Could you check a few things on this model? Use its own coordinates, in mm. Coordinates: 2 decimals unless noted, no trailing zeros. Write each loop counter-clockwise with the first axis right and the second up, starting at its lowest first coordinate (ties: lowest second). Pieces come first, ordered by that corner, then holes. Notation, with made-up numbers: M 10,-37.75 L 40,-37.75 A34 cw 40,-1.75 Z; hole C -15,-18.75 d8. An arc over 180 degrees is marked long. Answer as CSV lines item,"result". Start each with the question number.
Item 1: We'd pull the mould along X, two halves only. Please class faces 1 (the flat face through (212, 0, -68)), 2 (the cylindrical face through (355.283, 1.014, -88.32)): +X half, -X half, draft (parallel to the pull), parting line (faces both ways), or undercut.
Item 2: If I drill on line 1 along Z through (x, y) = (423, 1.1); line 2 along X through (y, z) = (0.7, -59); line 3 along Z through (x, y) = (338, 0.25), over which ranges is the centre line in solid material (lowest first)? Write a range as [from, to].
Item 3: Suppose I cut it at D-D, the plane x = 391. Write out the boundary of the cut face in (y, z), and give its area (3 significant figures).
Item 4: I'm going to push flat-ended pins straight in: P1, Ø6.5, axis at x = 7, z = -59, coming from the -Y side; P2, Ø1, axis at x = 5.5, y = 1, coming from the -Z side; P3, Ø0.6, axis at y = 1.5, z = -126.5, coming from the +X side; P4, Ø0.6, axis at x = 16.5, y = 1, coming from the +Z side. Where does each tip first touch, or does it pass through?
Item 5: Suppose I cut it at B-B, the plane z = -101. Write out the boundary of the cut face in (x, y).
Item 6: Suppose I cut it at C-C, the plane y = 0.4. Write out the boundary of the cut face in (x, z), and give its area (3 significant figures).
Item 7: Suppose I cut it at A-A, the plane x = 330. Write out the boundary of the cut face in (y, z).
```python
from build123d import *

# Parameters (mm, degrees)
SKETCH_2_W          = 430
SKETCH_2_H          = 135
EXTRUDE_1_DEPTH     = 2
SKETCH_3_R          = 2.5
SKETCH_3_W          = 12
SKETCH_3_H          = 15
SKETCH_3_W_2        = 60
SKETCH_3_H_2        = 30
CUT_EXTRUDE_1_DEPTH = 451.698347013
SKETCH_4_R          = 25.5
CUT_EXTRUDE_2_DEPTH = 451.698347013


with BuildPart() as part:
    # Эскиз2 → Бобышка-Вытянуть1 (new body)
    with BuildSketch(Plane(origin=(0, 0, 0), x_dir=(1, 0, 0), z_dir=(0, 1, 0))):
        with Locations((215, 67.5)):
            Rectangle(SKETCH_2_W, SKETCH_2_H)
    extrude(amount=EXTRUDE_1_DEPTH)

    # Эскиз3 → Вырез-Вытянуть1 (cut, through all)
    with BuildSketch(Plane(origin=(0, 2, 0), x_dir=(1, 0, 0), z_dir=(0, 1, 0))):
        with Locations(Location((7, 109, 0), (0, 0, 270))):
            Circle(SKETCH_3_R)
        with Locations(Location((423, 109, 0), (0, 0, 90))):
            Circle(SKETCH_3_R)
        with Locations(Location((7, 59, 0), (0, 0, 270))):
            Circle(SKETCH_3_R)
        with Locations(Location((423, 59, 0), (0, 0, 90))):
            Circle(SKETCH_3_R)
        with Locations((424, 127.5)):
            Rectangle(SKETCH_3_W, SKETCH_3_H)
        with Locations((6, 127.5)):
            Rectangle(SKETCH_3_W, SKETCH_3_H)
        with Locations((400, 15)):
            Rectangle(SKETCH_3_W_2, SKETCH_3_H_2)
        with Locations((30, 15)):
            Rectangle(SKETCH_3_W_2, SKETCH_3_H_2)
    extrude(amount=-CUT_EXTRUDE_1_DEPTH, mode=Mode.SUBTRACT)

    # Эскиз4 → Вырез-Вытянуть2 (cut, through all)
    with BuildSketch(Plane(origin=(0, 2, 0), x_dir=(1, 0, 0), z_dir=(0, 1, 0))):
        with Locations(Location((330, 85, 0), (0, 0, 270))):
            Circle(SKETCH_4_R)
    extrude(amount=-CUT_EXTRUDE_2_DEPTH, mode=Mode.SUBTRACT)


solid = part.part
```
Ans:
1,face 1,"draft"
1,face 2,"undercut"
2,line 1,"z = [-120, -111.5], [-106.5, -61.5], [-56.5, -30]"
2,line 2,"x = [0, 4.5], [9.5, 420.5], [425.5, 430]"
2,line 3,"z = [-135, -109.21], [-60.79, 0]"
3,outline,"M 0,-135 L 2,-135 L 2,-30 L 0,-30 Z"
3,area,"210 mm^2"
4,P1,"stops at y = 0"
4,P2,"stops at z = -120"
4,P3,"stops at x = 418"
4,P4,"stops at z = -30"
5,outline,"M 0,0 L 310.14,0 L 310.14,2 L 0,2 Z; M 349.86,0 L 430,0 L 430,2 L 349.86,2 Z"
6,outline,"M 0,-120 L 12,-120 L 12,-135 L 418,-135 L 418,-120 L 430,-120 L 430,-30 L 370,-30 L 370,0 L 60,0 L 60,-30 L 0,-30 Z; hole C 7,-109 d5; hole C 7,-59 d5; hole C 330,-85 d51; hole C 423,-109 d5; hole C 423,-59 d5"
6,area,"52,000 mm^2"
7,outline,"M 0,-135 L 2,-135 L 2,-110.5 L 0,-110.5 Z; M 0,-59.5 L 2,-59.5 L 2,0 L 0,0 Z"
